Design review of the part built by this model. Coordinates are the model's own, in mm. Face numbers are marked on the shaded views. A direction names the side the tool comes from. Give positions to 0.01 mm unless a question says otherwise; leave off trailing zeros. Order: outer loops, then holes, each group sorted by start corner. A loop starts at its lowest first (then second) coordinate and runs counter-clockwise, first axis right, second up. Notation, with made-up numbers: (51, -27) -> (83, -27) arc R20 cw to (83, -6) -> close; hole circle Ø11 at (-9, 2). An arc over 180 degrees is marked (long way). Return JSON: item names as keys, results as strings.
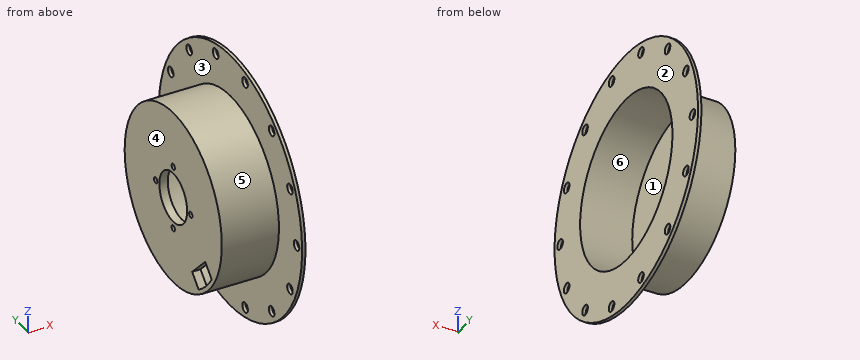
Autodesk Inventor part; units mm, degrees
ref_plane "YZ Plane" through (0, 0, 0) normal (1, 0, 0) x (0, 1, 0)
ref_plane "XZ Plane" through (0, 0, 0) normal (0, 1, 0) x (-1, 0, 0)
ref_plane "XY Plane" through (0, 0, 0) normal (0, 0, 1) x (1, 0, 0)
sketch "Sketch1" plane through (0, 0, 0) normal (1, 0, 0) x (0, 1, 0)
  circle A0 centre (0, 0) radius 19
  circle A1 centre (0, -19) radius 1.75
  circle A2 centre (19, 0) radius 1.75
  circle A3 centre (0, 19) radius 1.75
  circle A4 centre (-19, 0) radius 1.75
  circle A5 centre (0, 0) radius 52.5
  circle A6 centre (0, 0) radius 40
  dimension "d0" = 38
  dimension "d1" = 3.5
  dimension "d4" = 360
  dimension "d6" = 105
  dimension "d7" = 80
extrude "Extrusion1" add sketch "Sketch1" along normal blind 5 contours A2 A0 A1 A4 A3 | A5 | A6
sketch "Sketch2" plane through (0, 0, 0) normal (-1, 0, 0) x (0, 0, 1)
  circle A0 centre (0, 0) radius 52.5
  circle A1 centre (0, 0) radius 49.875
  dimension "d10" = 105
extrude "Extrusion2" add sketch "Sketch2" against normal blind 36
sketch "Sketch4" plane through (5, 0, 0) normal (1, 0, 0) x (0, 0, -1)
  circle A0 centre (0, 0) radius 15
  line L0 (0, 0) -> (7.0711, 7.0711)
  line L1 (0, 0) -> (10, 0) construction
  line L2 (7.0711, 7.0711) -> (41.6219, -27.4797)
  circle A1 centre (0, 0) radius 49.875
  line L3 (0, 0) -> (-7.0711, -7.0711)
  line L4 (-7.0711, -7.0711) -> (27.4797, -41.6219)
  line L5 (41.6219, -27.4797) -> (34.5508, -20.4087)
  line L6 (34.5508, -20.4087) -> (20.4087, -34.5508)
  point P0 (0.8346, -14.9768)
  point P1 (14.9768, -0.8346)
  point P2 (-49.875, 0)
  point P3 (-49.875, 0)
  dimension "d27" = 30
  dimension "d28" = 10
  dimension "d29" = 45
  dimension "d30" = 10
  dimension "d34" = 10
extrude "Extrusion4" cut sketch "Sketch4" against normal blind 10 contours A0 L2 L0 L3 L4 | L4 L3 L0 L2 A0 | L6 L2 A1 L4
sketch "Sketch6" plane through (36, 0, 0) normal (1, 0, 0) x (0, 0, -1)
  circle A0 centre (0, 0) radius 71.5
  circle A1 centre (0, 71.5) radius 3
  circle A2 centre (-55.901, 44.5795) radius 3
  circle A3 centre (-69.7073, -15.9102) radius 3
  circle A4 centre (-31.0227, -64.4193) radius 3
  circle A5 centre (31.0227, -64.4193) radius 3
  circle A6 centre (69.7073, -15.9102) radius 3
  circle A7 centre (55.901, 44.5795) radius 3
  circle A8 centre (0, 0) radius 15
  circle A9 centre (0, 0) radius 77.5
  circle A10 centre (0, 0) radius 49.875
  circle A11 centre (-31.0227, 64.4193) radius 3
  circle A12 centre (-55.901, 44.5795) radius 3
  circle A13 centre (-69.7073, 15.9102) radius 3
  circle A14 centre (-69.7073, -15.9102) radius 3
  circle A15 centre (-55.901, -44.5795) radius 3
  circle A16 centre (-31.0227, -64.4193) radius 3
  circle A17 centre (0, -71.5) radius 3
  circle A18 centre (31.0227, -64.4193) radius 3
  circle A19 centre (55.901, -44.5795) radius 3
  circle A20 centre (69.7073, -15.9102) radius 3
  circle A21 centre (69.7073, 15.9102) radius 3
  circle A22 centre (55.901, 44.5795) radius 3
  circle A23 centre (31.0227, 64.4193) radius 3
  dimension "d35" = 143
  dimension "d36" = 6
  dimension "d39" = 360
  dimension "d41" = 155
  dimension "d46" = 360
extrude "Extrusion6" add sketch "Sketch6" against normal blind 2 contours A0 A6 A19 A5 A17 A4 A15 A3 A13 A2 A11 A1 A23 A7 A21 | A9
equation "\"GapSize\" = Thickness"
equation "\"BendRadius\" = Thickness"
equation "\"MinimumRemnant\" = 2 * Thickness"
equation "\"BendReliefDepth\" = 0.5 * Thickness"
equation "\"BendReliefWidth\" = Thickness"
equation "\"CornerReliefSize\" = 4 * Thickness"
equation "\"JacobiRadiusSize\" = BendRadius"
equation "\"TransitionRadius\" = BendRadius"
properties part number "MotorCycDriveMount"
Item 1: Add section A-A (y = -25). Give the boundary of the cut face in (x, z), plus the area to 3 significant figures.
Result set:
{"outline": "(0, -46.17) -> (34, -46.17) -> (34, -73.36) -> (36, -73.36) -> (36, -43.16) -> (5, -43.16) -> (5, -39.14) -> (0, -39.14) -> close; (0, -29.96) -> (5, -29.96) -> (5, 43.16) -> (36, 43.16) -> (36, 73.36) -> (34, 73.36) -> (34, 46.17) -> (0, 46.17) -> close", "area": "711 mm^2"}
Item 2: Mouldability with a two-part tool opening along Z and no side actions: class the marked faces 4, 5 and 6 as released by +Z, released by -Z, zero draft, split by the parting line, or undercut.
Result set:
{"face 4": "zero draft", "face 5": "split by the parting line", "face 6": "undercut"}
Item 3: For pin 1 (4 mm diameter, centred on x = 23.5, z = 47, fed in from +Y); pin 2 (2 mm diameter, centred on x = 6, z = 24.5, fed in from +Y); pin 3 (9.5 mm diameter, centred on y = 15.91, z = 69.71, fed in from -X), all flat-tipped, find the tip position at first contact; note any pin that passes through.
Result set:
{"pin 1": "stops at y = 27.04", "pin 2": "stops at y = 46.95", "pin 3": "stops at x = 34"}
Item 4: Add section C-C (x = 12). Give the boundary of the cut face in (y, z) (3 decimals), plus the area to 3 significant figures.
Result set:
{"outline": "circle Ø105 at (0, 0); hole circle Ø99.75 at (0, 0)", "area": "844 mm^2"}
Item 5: Add section B-B (z = 55.5). Give the boundary of the cut face in (x, y).
Result set:
{"outline": "(34, -54.09) -> (36, -54.09) -> (36, -47.55) -> (34, -47.55) -> close; (34, -41.61) -> (36, -41.61) -> (36, 41.61) -> (34, 41.61) -> close; (34, 47.55) -> (36, 47.55) -> (36, 54.09) -> (34, 54.09) -> close"}
Item 6: Wall thickness on L1, parallel to Z at x = 1.5, y = 0; L2, parallel to Z at x = 28, y = 0 (3 decimals); L3, parallel to Y at x = 31, z = 28.5: over which ranges is each line inside the solid? List them lowest first. Write a range as [from, to].
Result set:
{"L1": "z = [-52.5, -20.75], [-17.25, -15], [15, 17.25], [20.75, 52.5]", "L2": "z = [-52.5, -49.875], [49.875, 52.5]", "L3": "y = [-44.09, -40.93], [40.93, 44.09]"}
Item 7: Machinability: for the marked faces 1, 2 and 3, which of the approach directions +Z, -Z, +X, -X, +Y, -Y give a long, thin tool a straight path to every point of the face, cutting with its end or side? Answer none if there is none.
Result set:
{"face 1": "+X", "face 2": "+Z, -Z, +X, +Y, -Y", "face 3": "-X"}
